Can you work these out from the model? Positions are in its coordinate system, mm. A direction names the side the tool comes from. Round coordinates to 2 decimals unless told otherwise and drop trailing zeros. Loops run counter-clockwise (first coordinate to the right, second up) from the corner with the lowest first, then second, coordinate; pieces in that order, holes last.
(1) I want a section at B-B on x = 86. Write out the boundary of the cut face in (y, z), plus the area to 3 significant figures.
(2) If I drill on line 1 along Y through (x, z) = (5, 2); line 2 along X through (y, z) = (1, 12); line 3 along Z through (x, y) = (62, 5.5), over which ranges is the centre line in solid material (lowest first)?
(3) Which directions (+Z, -Z, +X, -X, +Y, -Y) give clear straight access to the entire face, cutting with the end or side of a thin tool? Please do faces 4 (the face through (-21, 10, 4)), 5 (the face through (-2, 0, 5)).
(4) Will these pins go through, and if not, where does the flat tip stop? pin 1 Ø4 at (x, y) = (-14.9, 4.95) entering from +Z; pin 2 Ø3 at (x, y) = (5, -4.95) entering from -Z.
(5) Thinking about a two-plate mould opening in X: for faces 1 (the face through (-130, 0, 22)), 2 (the face through (135, 0, 20)), 3 (the face through (-2, 0, 0)), which applies, released by +X, released by -X, zero draft, split by the parting line, or undercut?
(6) I want a section at A-A on z = 14. Write out the boundary of the cut face in (x, y).
from build123d import *

# Parameters (mm, degrees)
SKETCH_1_W          = 270
SKETCH_1_H          = 20
EXTRUDE_1_DEPTH     = 5
SKETCH_2_W          = 5
SKETCH_2_H          = 20
EXTRUDE_2_DEPTH     = 35
SKETCH_3_W          = 5
SKETCH_3_H          = 20
EXTRUDE_3_DEPTH     = 35
SKETCH_4_R          = 1.6
CUT_EXTRUDE_1_DEPTH = 35
CUT_EXTRUDE_2_DEPTH = 274.130005675
SKETCH_6_R          = 1.5
CUT_EXTRUDE_3_DEPTH = 274.130005675


with BuildPart() as part:
    # 草图1 → 凸台-拉伸1 (new body)
    with BuildSketch(Plane.XY):
        Rectangle(SKETCH_1_W, SKETCH_1_H)
    extrude(amount=EXTRUDE_1_DEPTH)

    # 草图2 → 凸台-拉伸2 (add)
    with BuildSketch(Plane.XY.offset(5)):
        with Locations((-132.5, 0)):
            Rectangle(SKETCH_2_W, SKETCH_2_H)
    extrude(amount=EXTRUDE_2_DEPTH)

    # 草图3 → 凸台-拉伸3 (add)
    with BuildSketch(Plane.XY.offset(5)):
        with Locations((132.5, 0)):
            Rectangle(SKETCH_3_W, SKETCH_3_H)
    extrude(amount=EXTRUDE_3_DEPTH)

    # 草图4 → 切除-拉伸1 (cut)
    with BuildSketch(Plane(origin=(0, 0, 0), x_dir=(-1, 0, 0), z_dir=(0, 0, -1))):
        with Locations((5, 4.95)):
            Circle(SKETCH_4_R)
        with Locations((14.9, 4.95)):
            Circle(SKETCH_4_R)
        with Locations(Location((-14.9, 4.95, 0), (0, 0, 180))):
            Circle(SKETCH_4_R)
        with Locations(Location((-5, 4.95, 0), (0, 0, 180))):
            Circle(SKETCH_4_R)
        with Locations(Location((14.9, -4.95, 0), (0, 0, 180))):
            Circle(SKETCH_4_R)
        with Locations(Location((5, -4.95, 0), (0, 0, 180))):
            Circle(SKETCH_4_R)
        with Locations((-5, -4.95)):
            Circle(SKETCH_4_R)
        with Locations((-14.9, -4.95)):
            Circle(SKETCH_4_R)
    extrude(amount=-CUT_EXTRUDE_1_DEPTH, mode=Mode.SUBTRACT)

    # 草图5 → 切除-拉伸2 (cut, through all)
    with BuildSketch(Plane(origin=(135, 0, 0), x_dir=(0, 0, -1), z_dir=(1, 0, 0))):
        with BuildLine():
            ThreePointArc((-40, 0), (-37.071067812, 7.071067812), (-30, 10))
            Line((-30, 10), (-40, 10))
            Line((-40, 10), (-40, 0))
        make_face()
        with BuildLine():
            ThreePointArc((-30, -10), (-37.071067812, -7.071067812), (-40, 0))
            Line((-40, 0), (-40, -10))
            Line((-40, -10), (-30, -10))
        make_face()
    extrude(amount=-CUT_EXTRUDE_2_DEPTH, mode=Mode.SUBTRACT)

    # 草图6 → 切除-拉伸3 (cut, through all)
    with BuildSketch(Plane.ZY.offset(135)):
        with BuildLine():
            ThreePointArc((31.5, -6), (31.060660172, -4.939339828), (30, -4.5))
            Line((30, -4.5), (30, -7.5))
            ThreePointArc((30, -7.5), (31.060660172, -7.060660172), (31.5, -6))
        make_face()
        with BuildLine():
            Line((30, -7.5), (30, -4.5))
            ThreePointArc((30, -4.5), (28.5, -6), (30, -7.5))
        make_face()
        with Locations((24, 0)):
            Circle(SKETCH_6_R)
        with Locations((36, 0)):
            Circle(SKETCH_6_R)
        with BuildLine():
            ThreePointArc((31.5, 6), (31.060660172, 7.060660172), (30, 7.5))
            Line((30, 7.5), (30, 4.5))
            ThreePointArc((30, 4.5), (31.060660172, 4.939339828), (31.5, 6))
        make_face()
        with BuildLine():
            Line((30, 4.5), (30, 7.5))
            ThreePointArc((30, 7.5), (28.5, 6), (30, 4.5))
        make_face()
    extrude(amount=-CUT_EXTRUDE_3_DEPTH, mode=Mode.SUBTRACT)


solid = part.part
Filled sheet:
1. outline: (-10, 0) - (10, 0) - (10, 5) - (-10, 5) - close
1. area: 100 mm2
2. line 1: y = -10 to -6.55, -3.35 to 3.35, 6.55 to 10
2. line 2: x = -135 to -130, 130 to 135
2. line 3: z = 0 to 5
3. face 4: +Z, -Z, +X, -X, +Y
3. face 5: +Z, +Y, -Y
4. pin 1: stops at z = 5
4. pin 2: passes through
5. face 1: undercut
5. face 2: released by +X
5. face 3: zero draft
6. outline: (-135, -10) - (-130, -10) - (-130, 10) - (-135, 10) - close; (130, -10) - (135, -10) - (135, 10) - (130, 10) - close
